Could you check a few things on this model? Use its own coordinates, in mm. A direction names the side the tool comes from. Give positions to 0.01 mm unless a question says otherwise; leave off trailing zeros. Order: outer loops, then holes, each group sorted by start corner. A loop starts at its lowest first (then second) coordinate and runs counter-clockwise, first axis right, second up. Notation, with made-up numbers: (13, -35.5) -> (52, -35.5) arc R26 ccw to (52, -18.5) -> close; hole circle Ø9 at (14.25, 12.5). An arc over 180 degrees is marked (long way). One line per item, written item: value.
```python
from build123d import *

# Parameters (mm, degrees)
BOX_W             = 6
BOX_H             = 19
BOX_DEPTH         = 10
CYLINDER001_R     = 9
CYLINDER001_DEPTH = 10
CYLINDER_R        = 12
CYLINDER_DEPTH    = 4


with BuildPart() as cubo:
    # Box → Box (new body)
    with BuildSketch(Plane(origin=(-3, -4, 3), x_dir=(1, 0, 0), z_dir=(0, 0, 1))):
        with Locations((3, 9.5)):
            Rectangle(BOX_W, BOX_H)
    extrude(amount=BOX_DEPTH)


with BuildPart() as obj1:
    # Cylinder001 → Cylinder001 (new body)
    with BuildSketch(Plane(origin=(0, -4, 3), x_dir=(1, 0, 0), z_dir=(0, 0, 1))):
        Circle(CYLINDER001_R)
    extrude(amount=CYLINDER001_DEPTH)


with BuildPart() as cut002:
    # Cylinder → Cylinder (new body)
    with BuildSketch(Plane(origin=(0, -4, 1), x_dir=(1, 0, 0), z_dir=(0, 0, 1))):
        Circle(CYLINDER_R)
    extrude(amount=CYLINDER_DEPTH)

    # Cut001: cut obj1
    add(obj1.part, mode=Mode.SUBTRACT)

    # Cut002: cut Cubo
    add(cubo.part, mode=Mode.SUBTRACT)


solid = cut002.part
```
1) Suppose I cut it at A-A, the plane y = -4. Write out the boundary of the cut face in (x, z).
Answer below:
outline: (-12, 1) -> (12, 1) -> (12, 5) -> (9, 5) -> (9, 3) -> (-9, 3) -> (-9, 5) -> (-12, 5) -> close
2) If I drill on line 1 along X through (y, z) = (-4, 4.05); line 2 along Z through (x, y) = (-0.75, -12.5); line 3 along Y through (x, z) = (0, 4.6), over which ranges is the centre line in solid material (lowest first)?
Answer below:
line 1: x = -12 to -9, 9 to 12
line 2: z = 1 to 3
line 3: y = -16 to -13
3) Suppose I cut it at D-D, the plane x = 0. Write out the boundary of the cut face in (y, z).
Answer below:
outline: (-16, 1) -> (8, 1) -> (8, 3) -> (-13, 3) -> (-13, 5) -> (-16, 5) -> close
4) Suppose I cut it at B-B, the plane x = -4.25. Write out the boundary of the cut face in (y, z), then the cut area to 3 significant figures.
Answer below:
outline: (-15.22, 1) -> (7.22, 1) -> (7.22, 5) -> (3.93, 5) -> (3.93, 3) -> (-11.93, 3) -> (-11.93, 5) -> (-15.22, 5) -> close
area: 58.0 mm2
5) For P1, Ø1, axis at x = -2.5, z = 3, coming from the -Y side; P2, Ø1.5, axis at y = 2.5, z = 3, coming from the -X side; P3, Ø1, axis at y = 6, z = 4, coming from the +X side, each with a flat end and sliding along its axis, tell me the tip position at first contact or that it passes through.
Answer below:
P1: stops at y = -15.83
P2: stops at x = -10.53
P3: stops at x = 7.33
6) Suppose I cut it at C-C, the plane z = 3.9. Write out the boundary of the cut face in (x, y), then the cut area to 3 significant figures.
Answer below:
outline: (-3, 4.49) -> (-3, 7.62) arc R12 ccw (long way) to (3, 7.62) -> (3, 4.49) arc R9 cw (long way) to start
area: 180 mm2
7) For faces 4 (the cylindrical face through (0, -13, 4)), 5 (the flat face through (-3, 6, 4)), 6 (the flat face through (9, -6, 5)), which set-ups out of +Z, -Z, +X, -X, +Y, -Y let a thin tool reach every point of the face, with its end or its side?
Answer below:
face 4: +Z
face 5: +Z, +Y
face 6: +Z, +X, -X, +Y, -Y
8) We'd pull the mould along X, two halves only. Please class faces 1 (the flat face through (0, -2, 3)), 2 (the flat face through (0, -4, 1)), 3 (the cylindrical face through (-2.601, -15.715, 2.972)): +X half, -X half, draft (parallel to the pull), parting line (faces both ways), or undercut.
Answer below:
face 1: undercut
face 2: draft
face 3: parting line
